Check sheet for the drawn part. Datum: minimum x, y, z corner. Units: mm. Round coordinates to 2 decimals unless told otherwise and drop trailing zeros. Write each loop counter-clockwise with the first axis right and the second up, starting at its lowest first coordinate (ties: lowest second). Pieces come first, ordered by that corner, then holes.
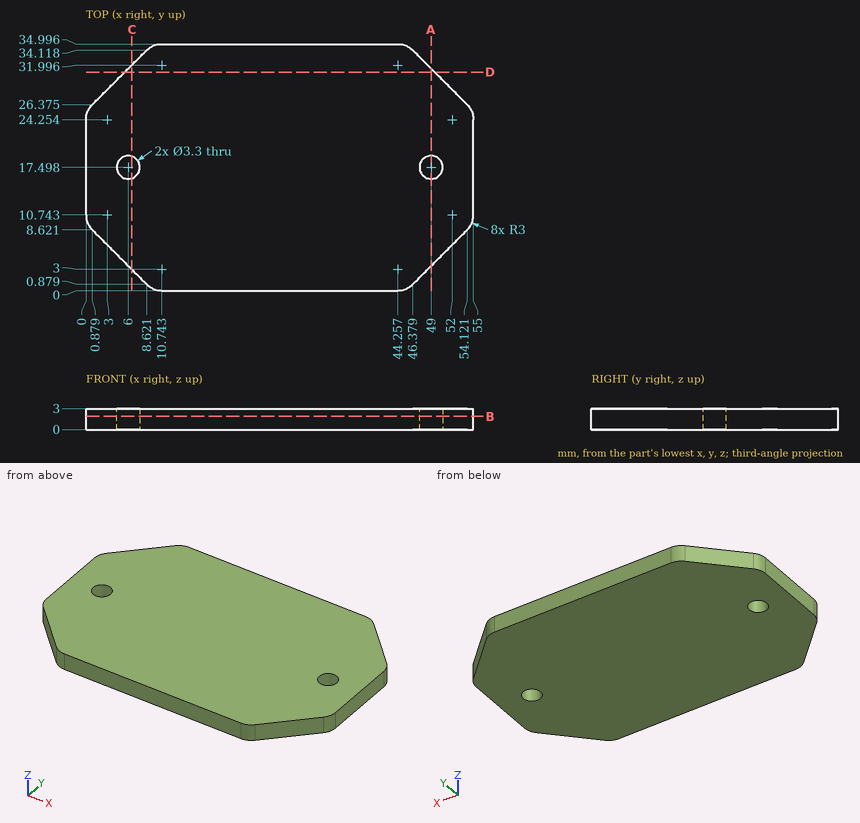
1. Go/stop test with a flat-tipped pin: pin 1 (3 mm diameter, centred on x = 48, y = 14, fed in from -Z). Record where the tip stops, or that it passes through.
2. Scan lines: line 1 along X through (y, z) = (24.5, 2.7); line 2 along Y through (x, z) = (50.5, 0.25) (1 decimal); line 3 along Y through (x, z) = (3, 1.55) (1 decimal). Record each from-to range of solid material in increasing order.
3. Sectioned sample at A-A, the plane x = 49. Enter the section's corners in (y, z).
4. Sectioned sample at B-B, the plane z = 1.9. Give the number of separate pieces and of enclosed holes in the cut face, plus the area to 3 significant figures.
5. Sectioned sample at C-C, the plane x = 6.5. Enter the section's corners in (y, z) (1 decimal).
6. Sectioned sample at D-D, the plane y = 31. Enter the section's corners in (x, z).
Computed values:
1. pin 1: stops at z = 0
2. line 1: x = 0.01 to 54.99
2. line 2: y = 5 to 16.8, 18.2 to 30
2. line 3: y = 6.5 to 28.5
3. outline: (3.5, 0) - (15.85, 0) - (15.85, 3) - (3.5, 3) - close; (19.15, 0) - (31.5, 0) - (31.5, 3) - (19.15, 3) - close
4. separate pieces: 1
4. enclosed holes: 2
4. area: 1,730 mm2
5. outline: (3, 0) - (15.9, 0) - (15.9, 3) - (3, 3) - close; (19.1, 0) - (32, 0) - (32, 3) - (19.1, 3) - close
6. outline: (5.5, 0) - (49.5, 0) - (49.5, 3) - (5.5, 3) - close
